from build123d import *

# Parameters (mm, degrees)
BOSS_EXTRUDE1_DEPTH = 25.2
SKETCH2_R           = 14
CUT_EXTRUDE1_DEPTH  = 25.2
SKETCH3_OUTSIDE_W   = 153.444
SKETCH3_OUTSIDE_H   = 160.946
SKETCH3_OUTSIDE_R   = 24.248711306
CUT_EXTRUDE2_DEPTH  = 25.2
CUT_EXTRUDE2_TAPER  = 60


with BuildPart() as part:
    # Sketch1 → Boss-Extrude1 (new body)
    with BuildSketch(Plane(origin=(0, 0, 0), x_dir=(0, 0, -1), z_dir=(1, 0, 0))):
        Polygon((0, 28), (-24.248711306, 14), (-24.248711306, -14), (0, -28), (24.248711306, -14), (24.248711306, 14), align=None)
    extrude(amount=-BOSS_EXTRUDE1_DEPTH)

    # Sketch2 → Cut-Extrude1 (cut)
    with BuildSketch(Plane(origin=(0, 0, 0), x_dir=(0, 0, -1), z_dir=(1, 0, 0))):
        Circle(SKETCH2_R)
    extrude(amount=-CUT_EXTRUDE1_DEPTH, mode=Mode.SUBTRACT)

    # Sketch3 outside → Cut-Extrude2 (cut)
    with BuildSketch(Plane(origin=(0, 0, 0), x_dir=(0, 0, -1), z_dir=(1, 0, 0))):
        Rectangle(SKETCH3_OUTSIDE_W, SKETCH3_OUTSIDE_H)
        Circle(SKETCH3_OUTSIDE_R, mode=Mode.SUBTRACT)
    extrude(amount=-CUT_EXTRUDE2_DEPTH, taper=CUT_EXTRUDE2_TAPER, mode=Mode.SUBTRACT)


solid = part.part
Build history of the part. All positions in model axes, mm. Coordinates: 2 decimals unless noted, no trailing zeros. Write each loop counter-clockwise with the first axis right and the second up, starting at its lowest first coordinate (ties: lowest second). Pieces come first, ordered by that corner, then holes. Notation, with made-up numbers: (-34.5, 76) -> (10.5, 76) arc R23 ccw to (10.5, 93) -> close; hole circle Ø2 at (56, 21). An arc over 180 degrees is marked (long way). Use CSV: the item, a comma, the result in double quotes. Start each with the question number.
Q1. Flat gauge pins, fed straight in: pin 1 Ø1.5 at (x, z) = (-22.5, -4) entering from -Y; pin 2 Ø10 at (x, y) = (-6, -20.5) entering from +Z; pin 3 Ø3 at (x, y) = (-3.5, 20.5) entering from +Z. Where does each tip first touch, or does it go through?
Q2. Cut at A-A, the plane x = -8. List the corners of the cut face in (y, z).
Q3. Pull direction Y, two halves, no side cores. Call faces 1 (the flat face through (-12.4, 20.9, -12.3)), 2 (the cylindrical face through (-12.424, -5.362, -12.932)), 3 (the conical face through (-0.526, -12.527, -21.82)): released by +Y, released by -Y, zero draft, split by the parting line, or undercut.
Q4. Drill centre lines: probe 1 along Y at (x, z) = (-6.75, 0); probe 2 along X at (y, z) = (-13, 20.5); probe 3 along Z at (x, y) = (-2.5, 2). Where is each one in solid material? Low to high.
Checked values:
1,pin 1,"stops at y = -26.12"
1,pin 2,"stops at z = 21.65"
1,pin 3,"stops at z = 15.59"
2,outline,"(-28, 0) -> (-14, -24.25) -> (14, -24.25) -> (28, 0) -> (14, 24.25) -> (-14, 24.25) -> close; hole circle Ø28 at (0, 0)"
3,face 1,"released by +Y"
3,face 2,"undercut"
3,face 3,"released by -Y"
4,probe 1,"y = -28 to -14, 14 to 28"
4,probe 2,"x = -25.2 to -0.01"
4,probe 3,"z = -24.25 to -13.86, 13.86 to 24.25"
